Check sheet for the modelled part. Datum: model origin and axes. Units: mm. A direction names the side the tool comes from. Give positions to 0.01 mm unless a question says otherwise; leave off trailing zeros. Loops run counter-clockwise (first coordinate to the right, second up) from the corner with the lowest first, then second, coordinate; pieces in that order, holes last. Notation, with made-up numbers: (75.5, -4.75) - (84.5, -4.75) arc R18 ccw to (84.5, 16.25) - close; hole circle Ø8 at (-12.75, -29.5). An arc over 180 degrees is marked (long way). Use CSV: the item, a comma, the result in double quotes.
from build123d import *

# Parameters (mm, degrees)
EXTRUDE_1_DEPTH     = 2
SKETCH_2_R          = 0.5
CUT_EXTRUDE_3_DEPTH = 2


with BuildPart() as part:
    # Эскиз1 → Бобышка-Вытянуть1 (new body)
    with BuildSketch(Plane.XY):
        with BuildLine():
            Line((33, -35), (-33, -35))
            ThreePointArc((-33, -35), (-34.414213562, -34.414213562), (-35, -33))
            Line((-35, -33), (-35, 33))
            ThreePointArc((-35, 33), (-34.414213562, 34.414213562), (-33, 35))
            Line((-33, 35), (33, 35))
            ThreePointArc((33, 35), (34.414213562, 34.414213562), (35, 33))
            Line((35, 33), (35, -33))
            ThreePointArc((35, -33), (34.414213562, -34.414213562), (33, -35))
        make_face()
        with BuildLine():
            Line((23, -25), (-23, -25))
            ThreePointArc((-23, -25), (-24.414213562, -24.414213562), (-25, -23))
            Line((-25, -23), (-25, 23))
            ThreePointArc((-25, 23), (-24.414213562, 24.414213562), (-23, 25))
            Line((-23, 25), (23, 25))
            ThreePointArc((23, 25), (24.414213562, 24.414213562), (25, 23))
            Line((25, 23), (25, -23))
            ThreePointArc((25, -23), (24.414213562, -24.414213562), (23, -25))
        make_face(mode=Mode.SUBTRACT)
    extrude(amount=EXTRUDE_1_DEPTH)

    # Эскиз2 → Вырез-Вытянуть3 (cut)
    with BuildSketch(Plane.XY):
        with Locations((-33, -0.5)):
            Circle(SKETCH_2_R)
    extrude(amount=CUT_EXTRUDE_3_DEPTH, mode=Mode.SUBTRACT)


solid = part.part
1. Sectioned sample at A-A, the plane x = -20.5. Record the boundary of the cut face in (y, z), and give its area (3 significant figures).
Completed:
outline,"(-35, 0) - (-25, 0) - (-25, 2) - (-35, 2) - close; (25, 0) - (35, 0) - (35, 2) - (25, 2) - close"
area,"40.0 mm²"
2. Sectioned sample at C-C, the plane z = 1.7. Record the boundary of the cut face in (x, y), and give its area (3 significant figures).
Completed:
outline,"(-35, -33) arc R2 ccw to (-33, -35) - (33, -35) arc R2 ccw to (35, -33) - (35, 33) arc R2 ccw to (33, 35) - (-33, 35) arc R2 ccw to (-35, 33) - close; hole circle Ø1 at (-33, -0.5); hole (-25, -23) arc R2 ccw to (-23, -25) - (23, -25) arc R2 ccw to (25, -23) - (25, 23) arc R2 ccw to (23, 25) - (-23, 25) arc R2 ccw to (-25, 23) - close"
area,"2,400 mm²"
3. Go/stop test with a flat-tipped pin: pin 1 Ø10 at (x, y) = (-8.5, -15.5) entering from -Z. Record where the tip stops, or that it passes through.
Completed:
pin 1,"passes through"
4. Release check for a two-part mould opening along X. For faces 1 (the face through (-24.43, 24.4, 0.99)), 2 (the face through (0, 35, 1)), 3 (the face through (-34.43, 34.4, 0.99)) record: released by +X, released by -X, zero draft, split by the parting line, or undercut.
Completed:
face 1,"undercut"
face 2,"zero draft"
face 3,"released by -X"
5. Scan lines: line 1 along Y through (x, z) = (8, 1.05); line 2 along Y through (x, z) = (-33, 1.6). Record each from-to range of solid material in increasing order.
Completed:
line 1,"y = -35 to -25, 25 to 35"
line 2,"y = -35 to -1, 0 to 35"
6. Set-up check for faces 4 (the face through (-25, 0, 1)), 5 (the face through (-35, 0, 1)): record each of +Z, -Z, +X, -X, +Y, -Y from which the full face is reachable in a straight line by a thin tool's end or side.
Completed:
face 4,"+Z, -Z"
face 5,"+Z, -Z, -X, +Y, -Y"
